Geometry check sheet. Reference: the model listing, model coordinates, mm. A direction names the side the tool comes from. Round coordinates to 2 decimals unless told otherwise and drop trailing zeros. Order: outer loops, then holes, each group sorted by start corner. A loop starts at its lowest first (then second) coordinate and runs counter-clockwise, first axis right, second up.
(1) Set-up check for faces 1 (the face through (0.03, 0.53, -12.57)), 2 (the face through (-1, 32.25, 2)), 3 (the face through (-27, -2, 2)), 4 (the face through (2, 0, -12)), 5 (the face through (-2, 0, -12)): record each of +Z, -Z, +X, -X, +Y, -Y from which the full face is reachable in a straight line by a thin tool's end or side.
(2) Cross-section at A-A on x = 32. Enter the section's corners in (y, z).
(3) Draft check along Y on faces 6 (the face through (-1, -32.25, 2)), 7 (the face through (-31.67, 29.23, 2.46)), 8 (the face through (-0.028, 25.373, -22.308)). Enter one of: pulls with the +Y half, pulls with the -Y half, needs draft (parallel to the pull), parting line crosses it, or undercut.
(4) Thickness scan on L1, parallel to X at y = 11, z = 1.5; L2, parallel to Y at x = 32, z = 3.3; L3, parallel to X at y = 26, z = 2. Record the ranges inside material, lowest first.
(5) Gauge pin test, flat ends, axial feed: P1, Ø5, axis at x = -4, z = -7.5, coming from the +Y side; P2, Ø22, axis at y = -2, z = -27.5, coming from the -X side; P3, Ø2, axis at x = 0.5, z = -27.5, coming from the +Y side. Record the tip position at first contact, or that the pin passes through.
(6) Cross-section at B-B on y = 0. Enter the section's corners in (x, z), and give its area (3 significant figures).
(7) Cross-section at C-C on y = -15.5. Enter the section's corners in (x, z), and give its area (3 significant figures).
(8) Cross-section at D-D on z = -14.5. Enter the section's corners in (x, y).
from build123d import *

# Parameters (mm, degrees)
SKETCH_1_W           = 75
SKETCH_1_H           = 64.5
EXTRUDE_1_DEPTH      = 5
EXTRUDE_2_DEPTH      = 2
EXTRUDE_2_DEPTH_BACK = 2
SKETCH_3_R           = 12
SKETCH_3_R_2         = 1.75
CUT_EXTRUDE_1_DEPTH  = 68.352152898
SKETCH_4_R           = 2.5
CUT_EXTRUDE_2_DEPTH  = 67.199037002
SKETCH_5_W           = 8
SKETCH_5_H           = 16
CUT_EXTRUDE_3_DEPTH  = 67.199037002


with BuildPart() as part:
    # 草圖1 → 填料-伸長1 (new body)
    with BuildSketch(Plane.XY):
        Rectangle(SKETCH_1_W, SKETCH_1_H)
    extrude(amount=EXTRUDE_1_DEPTH)

    # 草圖2 → 填料-伸長2 (add, two sides: drawn at the far end of the back side and taken through both)
    with BuildSketch(Plane(origin=(0, 0, 0), x_dir=(0, 0, -1), z_dir=(1, 0, 0)).offset(-EXTRUDE_2_DEPTH_BACK)):
        Polygon((0, 29.870222578), (0, 0), (0, -29.870222578), (44, -21), (44, 21), align=None)
    extrude(amount=EXTRUDE_2_DEPTH + EXTRUDE_2_DEPTH_BACK)

    # 草圖3 → 除料-伸長1 (cut, through all)
    with BuildSketch(Plane(origin=(2, 0, 0), x_dir=(0, 0, -1), z_dir=(1, 0, 0))):
        with Locations((24.559599052, 0)):
            Circle(SKETCH_3_R)
        with Locations((9.059599052, 15.5)):
            Circle(SKETCH_3_R_2)
        with Locations((40.059599052, 15.5)):
            Circle(SKETCH_3_R_2)
        with Locations((40.059599052, -15.5)):
            Circle(SKETCH_3_R_2)
        with Locations((9.059599052, -15.5)):
            Circle(SKETCH_3_R_2)
    extrude(amount=-CUT_EXTRUDE_1_DEPTH, mode=Mode.SUBTRACT)

    # 草圖4 → 除料-伸長2 (cut, through all)
    with BuildSketch(Plane(origin=(0, 0, 0), x_dir=(-1, 0, 0), z_dir=(0, 0, -1))):
        with Locations((32, 26.75)):
            Circle(SKETCH_4_R)
        with Locations(Location((32, -26.75, 0), (0, 0, 180))):
            Circle(SKETCH_4_R)
        with Locations((-32, -26.75)):
            Circle(SKETCH_4_R)
        with Locations(Location((-32, 26.75, 0), (0, 0, 180))):
            Circle(SKETCH_4_R)
    extrude(amount=-CUT_EXTRUDE_2_DEPTH, mode=Mode.SUBTRACT)

    # 草圖5 → 除料-伸長3 (cut, through all)
    with BuildSketch(Plane(origin=(0, 0, 0), x_dir=(-1, 0, 0), z_dir=(0, 0, -1))):
        with Locations((-27, 10)):
            Rectangle(SKETCH_5_W, SKETCH_5_H)
        with Locations((-27, -10)):
            Rectangle(SKETCH_5_W, SKETCH_5_H)
        with Locations((27, -10)):
            Rectangle(SKETCH_5_W, SKETCH_5_H)
        with Locations((27, 10)):
            Rectangle(SKETCH_5_W, SKETCH_5_H)
    extrude(amount=-CUT_EXTRUDE_3_DEPTH, mode=Mode.SUBTRACT)


solid = part.part
Found:
1. face 1: +X, -X
1. face 2: +Z, -Z, +X, -X, +Y
1. face 3: +Z, -Z
1. face 4: -Z, +X, +Y, -Y
1. face 5: -Z, -X, +Y, -Y
2. outline: (-32.25, 0) - (-29.25, 0) - (-29.25, 5) - (-32.25, 5) - close; (-24.25, 0) - (24.25, 0) - (24.25, 5) - (-24.25, 5) - close; (29.25, 0) - (32.25, 0) - (32.25, 5) - (29.25, 5) - close
3. face 6: pulls with the -Y half
3. face 7: undercut
3. face 8: pulls with the +Y half
4. L1: x = -37.5 to -31, -23 to 23, 31 to 37.5
4. L2: y = -32.25 to -29.25, -24.25 to 24.25, 29.25 to 32.25
4. L3: x = -37.5 to -34.38, -29.62 to 29.62, 34.38 to 37.5
5. P1: stops at y = 28.66
5. P2: stops at x = -2
5. P3: stops at y = 24.53
6. outline: (-37.5, 0) - (-2, 0) - (-2, -12.56) - (2, -12.56) - (2, 0) - (37.5, 0) - (37.5, 5) - (-37.5, 5) - close; (-2, -44) - (2, -44) - (2, -36.56) - (-2, -36.56) - close
6. area: 455 mm2
7. outline: (-37.5, 0) - (-31, 0) - (-31, 5) - (-37.5, 5) - close; (-23, 0) - (-2, 0) - (-2, -7.31) - (2, -7.31) - (2, 0) - (23, 0) - (23, 5) - (-23, 5) - close; (-2, -44) - (2, -44) - (2, -41.81) - (-2, -41.81) - close; (-2, -38.31) - (2, -38.31) - (2, -10.81) - (-2, -10.81) - close; (31, 0) - (37.5, 0) - (37.5, 5) - (31, 5) - close
7. area: 443 mm2
8. outline: (-2, -26.95) - (2, -26.95) - (2, -6.54) - (-2, -6.54) - close; (-2, 6.54) - (2, 6.54) - (2, 26.95) - (-2, 26.95) - close
